Verification items for the finished model (mm, model axes). Face numbers are marked on the shaded views. A direction names the side the tool comes from. Give positions to 0.01 mm unless a question says otherwise; leave off trailing zeros. Loops run counter-clockwise (first coordinate to the right, second up) from the corner with the lowest first, then second, coordinate; pieces in that order, holes last. Notation, with made-up numbers: (48.5, 62.5) - (69.5, 62.5) arc R20 cw to (69.5, 83.5) - close; hole circle Ø7 at (34, 39). An arc over 180 degrees is marked (long way). Use one line per item in the form item = value.
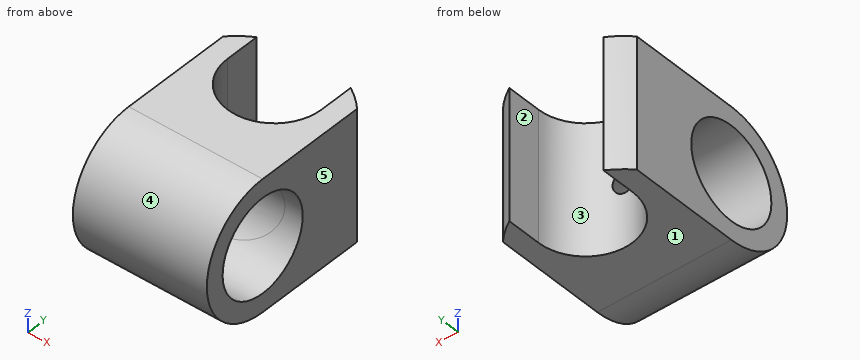
```python
from build123d import *
from build123d.topology import SkipClean

# Parameters (mm, degrees)
BODY_SPAR_LINK_DEPTH                               = 8.85
SKETCH2_R                                          = 6.35
WING_SPAR_EXTRUDE_DEPTH                            = 9.05
SMALL_CUT_COMPLETION_REACH                         = 24.706
SKETCH3_W                                          = 0.352155439
SKETCH3_H                                          = 17.7
CUT_CLEANUP_DEPTH                                  = 30.172161479
CUT_CLEANUP_DEPTH_BACK                             = 30.172161479
SKETCH4_R                                          = 6.35
EDGE_ROUNDING_TO_FIT_END_CAP_OF_FUSELAG_DEPTH      = 30.172161479
EDGE_ROUNDING_TO_FIT_END_CAP_OF_FUSELAG_DEPTH_BACK = 30.172161479
WING_SPAR_CUT_CLEANUP_DEPTH                        = 30.355663941
WING_SPAR_CUT_CLEANUP_DEPTH_BACK                   = 30.355663941
SKETCH6_R                                          = 6.35


with BuildPart() as part:
    # Sketch1 → Body spar link (new, symmetric)
    with BuildSketch(Plane.XY):
        with BuildLine():
            Line((-6.35, 0), (-6.35, 5.93510313))
            add(Edge.make_bspline(
                [(-6.35, 5.93510313), (-7.712058184, 5.755612708), (-9.05, 5.499803523)],
                knots=[1.753235264, 1.753235264, 1.753235264, 1.832339372, 1.832339372, 1.832339372], degree=2, weights=[1, 0.999217919, 1]))
            Line((-9.05, 5.499803523), (-9.05, 0))
            ThreePointArc((-9.05, 0), (0, -9.05), (9.05, 0))
            Line((9.05, 0), (9.05, 5.499803523))
            add(Edge.make_bspline(
                [(9.05, 5.499803523), (7.712058184, 5.755612708), (6.35, 5.93510313)],
                knots=[4.450845935, 4.450845935, 4.450845935, 4.529950043, 4.529950043, 4.529950043], degree=2, weights=[1, 0.999217919, 1]))
            Line((6.35, 5.93510313), (6.35, 0))
            ThreePointArc((6.35, 0), (0, -6.35), (-6.35, 0))
        make_face()
    extrude(amount=BODY_SPAR_LINK_DEPTH, both=True)

    # Sketch2 → Wing spar extrude (add, symmetric)
    with BuildSketch(Plane(origin=(0, 0, 0), x_dir=(0, 0, -1), z_dir=(1, 0, 0))):
        with BuildLine():
            Line((-8.85, -12.5), (-8.85, -2.5))
            Line((-8.85, -2.5), (8.85, -2.5))
            Line((8.85, -2.5), (8.85, -12.5))
            ThreePointArc((8.85, -12.5), (0, -21.35), (-8.85, -12.5))
        make_face()
        with Locations((0, -12.5)):
            Circle(SKETCH2_R, mode=Mode.SUBTRACT)
    extrude(amount=WING_SPAR_EXTRUDE_DEPTH, both=True)

    # Sketch3 → Small cut completion (add, up to next)
    with BuildSketch(Plane(origin=(0, -2.5, 0), x_dir=(1, 0, 0), z_dir=(0, 1, 0)), mode=Mode.PRIVATE) as small_cut_completion_sk1:
        with Locations((8.873922281, 0)):
            Rectangle(SKETCH3_W, SKETCH3_H)
    small_cut_completion_tool1 = extrude(small_cut_completion_sk1.sketch, amount=SMALL_CUT_COMPLETION_REACH, mode=Mode.PRIVATE) - part.part
    # Sketch3 → Small cut completion (add, up to next)
    with BuildSketch(Plane(origin=(0, -2.5, 0), x_dir=(1, 0, 0), z_dir=(0, 1, 0)), mode=Mode.PRIVATE) as small_cut_completion_sk2:
        with Locations((-8.873922281, 0)):
            Rectangle(SKETCH3_W, SKETCH3_H)
    small_cut_completion_tool2 = extrude(small_cut_completion_sk2.sketch, amount=SMALL_CUT_COMPLETION_REACH, mode=Mode.PRIVATE) - part.part
    add(small_cut_completion_tool1.solids().sort_by_distance((8.873922, -2.5, 0))[0])
    add(small_cut_completion_tool2.solids().sort_by_distance((-8.873922, -2.5, 0))[0])

    # Sketch4 → Cut cleanup (cut, two sides: drawn at the far end of the back side and taken through both)
    with SkipClean():  # the faces are left unmerged after this step: merging them gives an invalid solid
        with BuildSketch(Plane(origin=(0, 0, -8.85), x_dir=(-1, 0, 0), z_dir=(0, 0, -1)).offset(-CUT_CLEANUP_DEPTH_BACK)):
            Circle(SKETCH4_R)
        extrude(amount=CUT_CLEANUP_DEPTH + CUT_CLEANUP_DEPTH_BACK, mode=Mode.SUBTRACT)

    # Sketch5 → Edge rounding (to fit end cap of fuselage) (cut, two sides: drawn at the far end of the back side and taken through both)
    with SkipClean():  # the faces are left unmerged after this step: merging them gives an invalid solid
        with BuildSketch(Plane(origin=(0, 0, -8.85), x_dir=(-1, 0, 0), z_dir=(0, 0, -1)).offset(-EDGE_ROUNDING_TO_FIT_END_CAP_OF_FUSELAG_DEPTH_BACK)):
            with BuildLine():
                Line((-12.5, -6.15), (-22.5, -6.15))
                ThreePointArc((-22.5, -6.15), (0, 16.35), (22.5, -6.15))
                Line((22.5, -6.15), (12.5, -6.15))
                ThreePointArc((12.5, -6.15), (0, 6.35), (-12.5, -6.15))
            make_face()
        extrude(amount=EDGE_ROUNDING_TO_FIT_END_CAP_OF_FUSELAG_DEPTH + EDGE_ROUNDING_TO_FIT_END_CAP_OF_FUSELAG_DEPTH_BACK, mode=Mode.SUBTRACT)

    # Sketch6 → Wing spar cut cleanup (cut, two sides: drawn at the far end of the back side and taken through both)
    with BuildSketch(Plane(origin=(9.05, 0, 0), x_dir=(0, 0, -1), z_dir=(1, 0, 0)).offset(-WING_SPAR_CUT_CLEANUP_DEPTH_BACK)):
        with Locations((0, -12.5)):
            Circle(SKETCH6_R)
    extrude(amount=WING_SPAR_CUT_CLEANUP_DEPTH + WING_SPAR_CUT_CLEANUP_DEPTH_BACK, mode=Mode.SUBTRACT)


solid = part.part
```
1. Section check D-D, the plane y = -8. Record the cut outline in (x, z), then the cut area to 3 significant figures.
Result set:
outline = (-9.05, -8.85) - (9.05, -8.85) - (9.05, -4.48) - (-9.05, -4.48) - close; (-9.05, 4.48) - (9.05, 4.48) - (9.05, 8.85) - (-9.05, 8.85) - close
area = 158 mm²
2. Tool access check on the marked faces 1 and 2. Record the directions out of +Z, -Z, +X, -X, +Y, -Y that give a thin tool (end or side, any length) a straight path to the whole face; none if there is none.
Result set:
face_1 = -Z, +X, -X, +Y, -Y
face_2 = +Z, -Z, +Y
3. Draft check along X on the marked faces 3, 4 and 5. Enter one of: released by +X, released by -X, zero draft, split by the parting line, or undercut.
Result set:
face_3 = undercut
face_4 = zero draft
face_5 = released by +X
4. Scan lines: probe 1 along X at (y, z) = (2.25, -6.25); probe 2 along Y at (x, z) = (0, 0); probe 3 along X at (y, z) = (-4, 7). Record each from-to range of solid material in increasing order.
Result set:
probe_1 = -9.05 to -6.35, 6.35 to 9.05
probe_2 = -21.35 to -18.85
probe_3 = -9.05 to -4.93, 4.93 to 9.05
5. Section check A-A, the plane y = -4.5. Record the cut outline in (x, z).
Result set:
outline = (-9.05, -8.85) - (-4.48, -8.85) - (-4.48, 8.85) - (-9.05, 8.85) - close; (4.48, -8.85) - (9.05, -8.85) - (9.05, 8.85) - (4.48, 8.85) - close
6. Section check C-C, the plane x = 5.25. Record the cut outline in (y, z), then the cut area to 3 significant figures.
Result set:
outline = (-12.5, -8.85) - (-3.57, -8.85) - (-3.57, 8.85) - (-12.5, 8.85) arc R8.85 ccw to start; hole circle Ø12.7 at (-12.5, 0)
area = 154 mm²
7. Section check B-B, the plane z = 0. Record the cut outline in (x, y).
Result set:
outline = (-9.05, -21.35) - (9.05, -21.35) - (9.05, -18.85) - (-9.05, -18.85) - close; (-9.05, -6.15) - (-1.58, -6.15) arc R6.35 cw to (-6.35, 0) - (-6.35, 4.62) arc R12.5 ccw to (-9.05, 2.47) - close; (1.58, -6.15) - (9.05, -6.15) - (9.05, 2.47) arc R12.5 ccw to (6.35, 4.62) - (6.35, 0) arc R6.35 cw to start
